For this review, use the dimensioned drawing (mm, ordinates from the lowest corner) and the shaded views. Round coordinates to 2 decimals unless told otherwise and drop trailing zeros. Loops run counter-clockwise (first coordinate to the right, second up) from the corner with the lowest first, then second, coordinate; pieces in that order, holes last. Notation, with made-up numbers: (68.25, 27.25) - (92.25, 27.25) arc R21 ccw to (92.25, 34.25) - close; hole circle Ø7 at (77, 74.5). An arc over 180 degrees is marked (long way). Return JSON: item names as keys, results as strings. Group by question number.
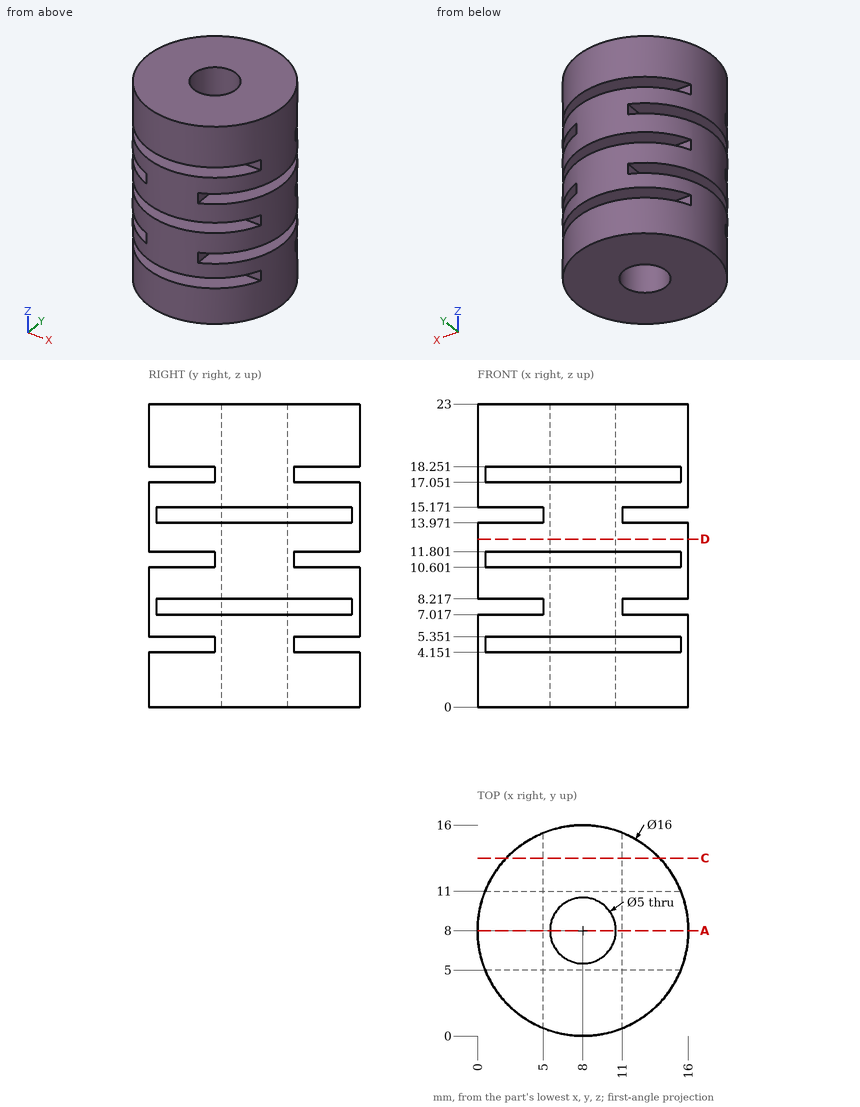
Q1. Add section C-C, the plane y = 13.5. Give the number of separate pieces and of enclosed holes in the cut face, plus the area to 3 significant figures.
Q2. Insertion check: pin 1 Ø8 at (x, z) = (1.5, 15) entering from -Y; pin 2 Ø2 at (x, z) = (3, 19.5) entering from +Y; pin 3 Ø2 at (y, z) = (6, 7.5) entering from -X. Each pin has a flat end and moves straight along its axis. Give the tip position at first contact, or say it passes through.
Q3. Add section D-D, the plane z = 12.75. State the section outline as (x, y) points, plus the area to 3 significant figures.
Q4. Add section A-A, the plane y = 8. State the section outline as (x, z) points, plus the area to 3 significant figures.
Q5. For line 1 (Z direction, x = 6.25, y = 3.5); line 2 (Z direction, x = 11.5, y = 7.75); line 3 (Y direction, x = 8, z = 5), list the stretches that pass through material, from the lowest coordinate up.
Evaluation:
{
 "1": {"separate pieces": "4", "enclosed holes": "0", "area": "212 mm²"},
 "2": {"pin 1": "y = 0.4", "pin 2": "y = 14.93", "pin 3": "x = 0.08"},
 "3": {"outline": "circle Ø16 at (8, 8); hole circle Ø5 at (8, 8)", "area": "181 mm²"},
 "4": {"outline": "(0, 0) - (5.5, 0) - (5.5, 23) - (0, 23) - (0, 15.17) - (5, 15.17) - (5, 13.97) - (0, 13.97) - (0, 8.22) - (5, 8.22) - (5, 7.02) - (0, 7.02) - close; (10.5, 0) - (16, 0) - (16, 7.02) - (11, 7.02) - (11, 8.22) - (16, 8.22) - (16, 13.97) - (11, 13.97) - (11, 15.17) - (16, 15.17) - (16, 23) - (10.5, 23) - close", "area": "229 mm²"},
 "5": {"line 1": "0 to 4.15, 5.35 to 10.6, 11.8 to 17.05, 18.25 to 23", "line 2": "0 to 7.02, 8.22 to 13.97, 15.17 to 23", "line 3": "5 to 5.5, 10.5 to 11"}
}
